```python
from build123d import *

# Parameters (mm, degrees)
F1_DEPTH = 22
F2_T     = -0.5
F3_R     = 1


with BuildPart() as f1:
    # F0 (on Top) → F1 (new body)
    with BuildSketch(Plane.XY):
        with BuildLine():
            ThreePointArc((0, 3), (0.8786796564, 0.8786796564), (3, 0))
            Line((3, 0), (42, 0))
            ThreePointArc((42, 0), (44.1213203436, 0.8786796564), (45, 3))
            Line((45, 3), (45, 22))
            ThreePointArc((45, 22), (44.1213203436, 24.1213203436), (42, 25))
            Line((42, 25), (3, 25))
            ThreePointArc((3, 25), (0.8786796564, 24.1213203436), (0, 22))
            Line((0, 22), (0, 3))
        make_face()
    extrude(amount=F1_DEPTH)

    # F2
    f2_openings = [f1.faces().sort_by_distance(p)[0] for p in [
        (22.5, 12.5, 22),
    ]]
    offset(amount=F2_T, openings=f2_openings)

    # F3
    f3_edges = [f1.edges().sort_by_distance(p)[0] for p in [
        (0.5, 12.5, 0.5),
        (1.232233, 1.232233, 0.5),
        (22.5, 0.5, 0.5),
        (43.767767, 1.232233, 0.5),
        (44.5, 12.5, 0.5),
        (43.767767, 23.767767, 0.5),
        (22.5, 24.5, 0.5),
        (1.232233, 23.767767, 0.5),
    ]]
    fillet(f3_edges, radius=F3_R)


solid = f1.part
```
Work out the finished part from the listing and answer in its coordinate system (mm). A direction names the side the tool comes from. Round coordinates to 2 decimals unless told otherwise and drop trailing zeros. Write each loop counter-clockwise with the first axis right and the second up, starting at its lowest first coordinate (ties: lowest second). Pieces come first, ordered by that corner, then holes.
1) A flat-ended cylindrical pin translates along its axis: P1, Ø2, axis at x = 37.5, y = 10, coming from the +Z side. Find the tip coordinate at first contact, or state that the pin passes through.
2) Determine the mould class of faces 1 (the face through (23, 25, 11)), 2 (the face through (0, 13, 11)), 3 (the face through (43.787, 23.748, 11.606)), 4 (the face through (22.227, 24.215, 0.801)) for opening direction X: pulls with the +X half, pulls with the -X half, needs draft (parallel to the pull), parting line crosses it, or undercut.
3) Which of the six approach directions +Z, -Z, +X, -X, +Y, -Y give full straight-line access (tool end or side, diameter ignored) to faces 5 (the face through (0.86, 0.9, 10.85)), 6 (the face through (0.785, 12.367, 0.801))?
4) Consider probe 1 along X at (y, z) = (9.5, 17.75); probe 2 along Y at (x, z) = (25, 3.25); probe 3 along Z at (x, y) = (4.5, 20). Determine where each line is inside the solid, lowest interval first.
5) A cutting plane is placed at A-A on z = 7.75. Determine the outline of the cut face in (x, y).
6) A cutting plane is placed at B-B on x = 25. Determine the outline of the cut face in (y, z), and give its area (3 significant figures).
7) A cutting plane is placed at C-C on y = 7. Determine the outline of the cut face in (x, z), and give its area (3 significant figures).
Entries:
1. P1: stops at z = 0.5
2. face 1: needs draft
2. face 2: pulls with the -X half
2. face 3: undercut
2. face 4: undercut
3. face 5: +Z, -Z, -X, -Y
3. face 6: +Z
4. probe 1: x = 0 to 0.5, 44.5 to 45
4. probe 2: y = 0 to 0.5, 24.5 to 25
4. probe 3: z = 0 to 0.5
5. outline: (0, 3) arc R3 ccw to (3, 0) - (42, 0) arc R3 ccw to (45, 3) - (45, 22) arc R3 ccw to (42, 25) - (3, 25) arc R3 ccw to (0, 22) - close; hole (0.5, 3) arc R2.5 ccw to (3, 0.5) - (42, 0.5) arc R2.5 ccw to (44.5, 3) - (44.5, 22) arc R2.5 ccw to (42, 24.5) - (3, 24.5) arc R2.5 ccw to (0.5, 22) - close
6. outline: (0, 0) - (25, 0) - (25, 22) - (24.5, 22) - (24.5, 1.5) arc R1 cw to (23.5, 0.5) - (1.5, 0.5) arc R1 cw to (0.5, 1.5) - (0.5, 22) - (0, 22) - close
6. area: 34.4 mm2
7. outline: (0, 0) - (45, 0) - (45, 22) - (44.5, 22) - (44.5, 1.5) arc R1 cw to (43.5, 0.5) - (1.5, 0.5) arc R1 cw to (0.5, 1.5) - (0.5, 22) - (0, 22) - close
7. area: 44.4 mm2
